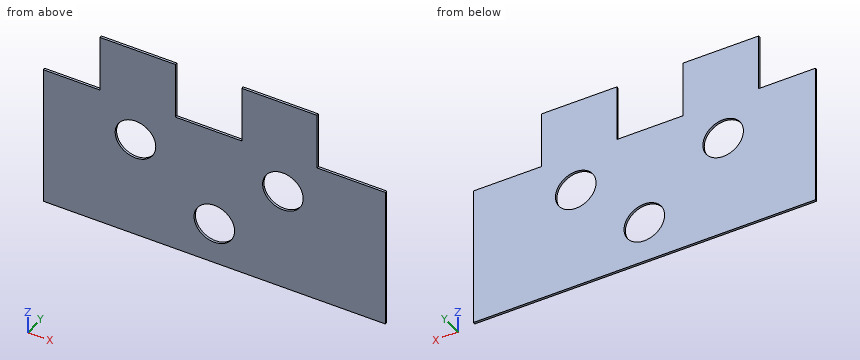
```python
from build123d import *

# Parameters (mm, degrees)
F0_W     = 13
F0_H     = 10
F0_R     = 3.5
F1_DEPTH = 0.2


with BuildPart() as f1:
    # F0 (on Front) → F1 (new body, symmetric)
    with BuildSketch(Plane.XZ):
        with Locations((-13.206897, 17.5)):
            Rectangle(F0_W, F0_H)
        Polygon((-19.706897, 12.5), (-29.5, 12.5), (-29.5, -12.5), (29.5, -12.5), (29.5, 12.5), (17.729655, 12.5), (4.729655, 12.5), (-6.706897, 12.5), align=None)
        with Locations((0, -5.123793)):
            Circle(F0_R, mode=Mode.SUBTRACT)
        with Locations((-13.597759, 5.517931)):
            Circle(F0_R, mode=Mode.SUBTRACT)
        with Locations((11.824138, 5.715)):
            Circle(F0_R, mode=Mode.SUBTRACT)
        with Locations((11.229655, 17.5)):
            Rectangle(F0_W, F0_H)
    extrude(amount=F1_DEPTH, both=True)


solid = f1.part
```
CAD build for the part. Positions are in the model's coordinates, mm. Round coordinates to 2 decimals unless told otherwise and drop trailing zeros. Loops run counter-clockwise (first coordinate to the right, second up) from the corner with the lowest first, then second, coordinate; pieces in that order, holes last. Notation, with made-up numbers: M 36.25,38 L 95.25,38 A17 ccw 95.25,60 Z; hole C -34.5,-9 d2. An arc over 180 degrees is marked long. Return JSON: item names as keys, results as strings. Group by question number.
(1) Drop a flat-ended pin along its axis: P1, Ø4, axis at x = 11.82, z = 5.72, coming from the -Y side. Give the stop position or say it passes through.
(2) Saw through at C-C, the plane x = 9. List the corners of the cut face in (y, z).
(3) Saw through at B-B, the plane y = -0.05. List the corners of the cut face in (x, z) (3 decimals), and give its area (3 significant figures).
(4) Saw through at A-A, the plane x = 0. List the corners of the cut face in (y, z), and give its area (3 significant figures).
(5) Saw through at D-D, the plane x = 18.5. List the corners of the cut face in (y, z), and give its area (3 significant figures).
(6) Wall check: probe 1 along X at (y, z) = (0.1, 17); probe 2 along X at (y, z) = (0, 8.5); probe 3 along X at (y, z) = (0.1, 4). Give the ranges that are in metal, low to high. Write a range as [from, to].
Answer list:
{
 "1": {"P1": "through"},
 "2": {"outline": "M -0.2,-12.5 L 0.2,-12.5 L 0.2,3.65 L -0.2,3.65 Z; M -0.2,7.78 L 0.2,7.78 L 0.2,22.5 L -0.2,22.5 Z"},
 "3": {"outline": "M -29.5,-12.5 L 29.5,-12.5 L 29.5,12.5 L 17.73,12.5 L 17.73,22.5 L 4.73,22.5 L 4.73,12.5 L -6.707,12.5 L -6.707,22.5 L -19.707,22.5 L -19.707,12.5 L -29.5,12.5 Z; hole C -13.598,5.518 d7; hole C 0,-5.124 d7; hole C 11.824,5.715 d7", "area": "1,620 mm2"},
 "4": {"outline": "M -0.2,-12.5 L 0.2,-12.5 L 0.2,-8.62 L -0.2,-8.62 Z; M -0.2,-1.62 L 0.2,-1.62 L 0.2,12.5 L -0.2,12.5 Z", "area": "7.20 mm2"},
 "5": {"outline": "M -0.2,-12.5 L 0.2,-12.5 L 0.2,12.5 L -0.2,12.5 Z", "area": "10.0 mm2"},
 "6": {"probe 1": "[-19.71, -6.71], [4.73, 17.73]", "probe 2": "[-29.5, -15.43], [-11.77, 9.7], [13.94, 29.5]", "probe 3": "[-29.5, -16.75], [-10.44, 8.77], [14.88, 29.5]"}
}
